Model file for the job. Use its own axes, mm. A direction names the side the tool comes from. Give positions to 0.01 mm unless a question says otherwise; leave off trailing zeros. Order: outer loops, then holes, each group sorted by start corner. A loop starts at its lowest first (then second) coordinate and runs counter-clockwise, first axis right, second up. Notation, with made-up numbers: (-29, 45) - (11, 45) arc R30 ccw to (11, 78) - close; hole circle Ø7 at (52.25, 34). An arc over 180 degrees is marked (long way). Use CSV: the item, a comma, the result in double quotes. Start each with the question number.
(1) Probe L1, parallel to X at y = 34.5, z = 16; L2, parallel to X at y = 8, z = 2; L3, parallel to Z at x = -49, y = 11.5. List the from-to ranges inside material, lowest first.
(2) Drop flat-ended pins along their axis: pin 1 Ø22.5 at (x, y) = (-44, 16) entering from +Z; pin 2 Ø2 at (y, z) = (27, 15) entering from -X; pin 3 Ø11.5 at (x, y) = (32, 14) entering from +Z; pin 4 Ø10.5 at (x, y) = (-41.98, 14.01) entering from +Z. Give the stop position or say it passes through.
(3) Band-saw the part on A-A, the plane z = 41. Give the cut face in (x, y), then the cut area to 3 significant figures.
(4) Band-saw the part on C-C, the plane y = 24. Give the cut face in (x, z).
(5) Band-saw the part on B-B, the plane x = -46. Give the cut face in (y, z).
(6) Band-saw the part on D-D, the plane x = 44.5. Give the cut face in (y, z).
(7) Pull direction Y, two halves, no side cores. Call faces 6 (the flat face through (6, 48, 19)), 7 (the cylindrical face through (-48.475, 14.294, 6.743)), 8 (the flat face through (47, 9, 49.168)): +Y half, -Y half, draft (parallel to the pull), parting line (faces both ways), or undercut.
(8) Tool access for faces 1 (the cylindrical face through (46.6, 23.9, 18.5)), 2 (the flat face through (34, 24, 13.299)), 3 (the cylindrical face through (-43.39, 29.663, 6.743)), 4 (the flat face through (-41, 24, 13.299)), 5 (the flat face through (47, 39, 49.168)): list every direction of +Z, -Z, +X, -X, +Y, -Y with a clear straight run to the whole face (end or side of a thin tool).
from build123d import *

# Parameters (mm, degrees)
F1_DEPTH = 48
F3_DEPTH = 11
F4_R     = 6.5
F5_DEPTH = 13.300004


with BuildPart() as f1:
    # F0 (on Front) → F1 (new body)
    with BuildSketch(Plane.XZ):
        with BuildLine():
            Line((-54.981197, 0), (-19, 0))
            ThreePointArc((-19, 0), (0, 19), (19, 0))
            Line((19, 0), (52.018803, 0))
            Line((52.018803, 0), (52.018803, 49.16832))
            Line((52.018803, 49.16832), (41.018803, 49.16832))
            Line((41.018803, 49.16832), (41.018803, 13.299004))
            Line((41.018803, 13.299004), (26.891197, 13.299004))
            ThreePointArc((26.891197, 13.299004), (0, 30), (-26.891197, 13.299004))
            Line((-26.891197, 13.299004), (-54.981197, 13.299004))
            Line((-54.981197, 13.299004), (-54.981197, 0))
        make_face()
    extrude(amount=-F1_DEPTH)

    # F2 (on face) → F3 (cut)
    with BuildSketch(Plane.YZ.offset(52.018803)):
        with BuildLine():
            Line((30.5, 49.16832), (17.5, 49.16832))
            Line((17.5, 49.16832), (17.5, 25))
            ThreePointArc((17.5, 25), (24, 18.5), (30.5, 25))
            Line((30.5, 25), (30.5, 49.16832))
        make_face()
    extrude(amount=-F3_DEPTH, mode=Mode.SUBTRACT)

    # F4 (on face) → F5 (cut, through all)
    with BuildSketch(Plane.XY.offset(13.299004)):
        with Locations((-41.981197, 36.00838)):
            Circle(F4_R)
        with Locations((-41.981197, 14.00838)):
            Circle(F4_R)
    extrude(amount=-F5_DEPTH, mode=Mode.SUBTRACT)


solid = f1.part
Answer block:
1,L1,"x = -25.38 to -10.25, 10.25 to 25.38, 41.02 to 52.02"
1,L2,"x = -54.98 to -44.46, -39.5 to -18.89, 18.89 to 52.02"
1,L3,"z = 0 to 13.3"
2,pin 1,"stops at z = 13.3"
2,pin 2,"stops at x = -26.53"
2,pin 3,"stops at z = 14.52"
2,pin 4,"passes through"
3,outline,"(41.02, 0) - (52.02, 0) - (52.02, 17.5) - (41.02, 17.5) - close; (41.02, 30.5) - (52.02, 30.5) - (52.02, 48) - (41.02, 48) - close"
3,area,"385 mm2"
4,outline,"(-54.98, 0) - (-19, 0) arc R19 cw to (19, 0) - (52.02, 0) - (52.02, 18.5) - (41.02, 18.5) - (41.02, 13.3) - (26.89, 13.3) arc R30 ccw to (-26.89, 13.3) - (-54.98, 13.3) - close"
5,outline,"(0, 0) - (8.9, 0) - (8.9, 13.3) - (0, 13.3) - close; (19.12, 0) - (30.9, 0) - (30.9, 13.3) - (19.12, 13.3) - close; (41.12, 0) - (48, 0) - (48, 13.3) - (41.12, 13.3) - close"
6,outline,"(0, 0) - (48, 0) - (48, 49.17) - (30.5, 49.17) - (30.5, 25) arc R6.5 cw to (17.5, 25) - (17.5, 49.17) - (0, 49.17) - close"
7,face 6,"+Y half"
7,face 7,"undercut"
7,face 8,"draft"
8,face 1,"+Z, +X"
8,face 2,"+Z, +Y, -Y"
8,face 3,"+Z, -Z"
8,face 4,"+Z, -X, +Y, -Y"
8,face 5,"+Z, +X, -X, +Y, -Y"
